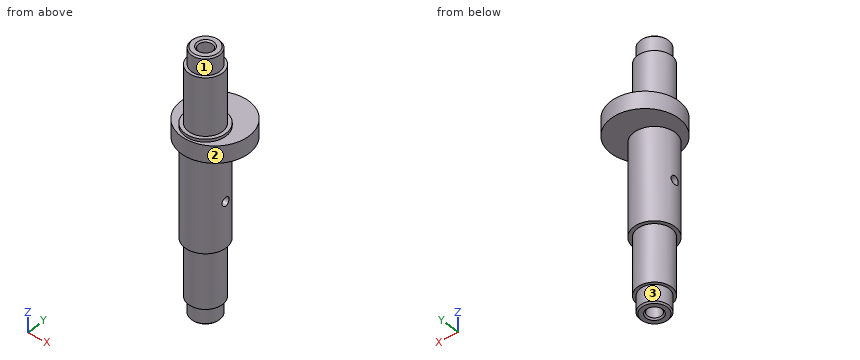
Autodesk Inventor part; units mm, degrees
ref_plane "YZ Plane" through (0, 0, 0) normal (1, 0, 0) x (0, 1, 0)
ref_plane "XZ Plane" through (0, 0, 0) normal (0, 1, 0) x (-1, 0, 0)
ref_plane "XY Plane" through (0, 0, 0) normal (0, 0, 1) x (1, 0, 0)
sketch "Sketch1" plane through (0, 0, 0) normal (0, 0, 1) x (1, 0, 0)
  circle A0 centre (0, 0) radius 12
  dimension "d0" = 24
extrude "Extrusion1" add sketch "Sketch1" along normal blind 92.4
sketch "Sketch2" plane through (0, 0, 92.4) normal (0, 0, 1) x (1, 0, 0)
  circle A0 centre (0, 0) radius 12
  circle A1 centre (0, 0) radius 5
  dimension "d3" = 10
extrude "Extrusion2" cut sketch "Sketch2" against normal blind 6.2
sketch "Sketch3" plane through (0, 0, 86.2) normal (0, 0, 1) x (1, 0, 0)
  circle A0 centre (0, 0) radius 12
  circle A1 centre (0, 0) radius 6
  dimension "d6" = 12
extrude "Extrusion3" cut sketch "Sketch3" against normal blind 20.2
sketch "Sketch4" plane through (0, 0, 66) normal (0, 0, 1) x (1, 0, 0)
  circle A0 centre (0, 0) radius 12
  circle A1 centre (0, 0) radius 7.25
  dimension "d9" = 14.5
extrude "Extrusion4" cut sketch "Sketch4" against normal blind 1
sketch "Sketch5" plane through (0, 0, 0) normal (0, 0, -1) x (-1, 0, 0)
  circle A0 centre (0, 0) radius 12
  circle A1 centre (0, 0) radius 6
  dimension "d12" = 0
  dimension "d13" = 12
extrude "Extrusion5" cut sketch "Sketch5" against normal blind 26.4
sketch "Sketch6" plane through (0, 0, 0) normal (0, 0, -1) x (-1, 0, 0)
  circle A0 centre (0, 0) radius 6
  circle A1 centre (0, 0) radius 5
  dimension "d16" = 10
extrude "Extrusion6" cut sketch "Sketch6" against normal blind 6.2
sketch "Sketch7" plane through (0, 0, 26.4) normal (0, 0, -1) x (-1, 0, 0)
  circle A0 centre (0, 0) radius 6
  circle A1 centre (0, 0) radius 12
  circle A2 centre (0, 0) radius 7.25
  dimension "d19" = 14.5
extrude "Extrusion7" cut sketch "Sketch7" against normal blind 32.6 contours A1
sketch "Sketch8" plane through (0, 0, 0) normal (0, 0, -1) x (-1, 0, 0)
  circle A0 centre (0, 0) radius 5
hole "Hole1" at (0, 0, 0) direction (0, 0, 1) diameter 4.917 depth 18 tip angle 118
chamfer "Chamfer1" distance 0.5 angle 45 1 edges at (0, -2.4585, 0)
sketch "Sketch9" plane through (0, 0, 92.4) normal (0, 0, 1) x (1, 0, 0)
  circle A0 centre (0, 0) radius 5
hole "Hole2" at (0, 0, 92.4) direction (0, 0, -1) diameter 4.917 depth 18 tip angle 118
chamfer "Chamfer2" distance 0.5 angle 45 1 edges at (0, 2.4585, 92.4)
chamfer "Chamfer3" distance 0.5 angle 45 2 edges at (-5, 0, 92.4) (5, 0, 0)
sketch "Sketch10" plane through (0, 0, 65) normal (0, 0, 1) x (1, 0, 0)
  circle A0 centre (0, 0) radius 7.25
  circle A1 centre (0, 4) radius 12
  dimension "d46" = 24
  dimension "d47" = 4
extrude "Extrusion8" add sketch "Sketch10" against normal blind 6
sketch "Sketch11" plane through (0, 0, 65) normal (0, 0, 1) x (1, 0, 0)
  arc A0 (-11.8322, 2) -> (11.8322, 2) centre (0, 0) ccw
  arc A1 (11.8322, 2) -> (-11.8322, 2) centre (0, 4) ccw
  circle A2 centre (0, 4) radius 12
extrude "Extrusion9" cut sketch "Sketch11" against normal blind 6 contours A2 A0
sketch "Sketch13" plane through (0, 0, 0) normal (1, 0, 0) x (0, 1, 0)
  circle A0 centre (0, 42.45) radius 1.5
  line L0 (-8, 59) -> (16, 59)
  line L1 (-7.25, 59) -> (7.25, 59)
  line L2 (-7.25, 26.4) -> (7.25, 26.4)
  point P0 (0, 0)
  dimension "d56" = 3
  dimension "d57" = 16.55
extrude "Extrusion11" cut sketch "Sketch13" along normal mid plane 20
properties part number "EIXO EXCÊNTRICO(53)" material "Carbon Steel"
Part model, mm, in its own coordinate system. Face numbers are marked on the shaded views. A direction names the side the tool comes from. Coordinates: 2 decimals unless noted, no trailing zeros. Loops run counter-clockwise (first coordinate to the right, second up) from the corner with the lowest first, then second, coordinate; pieces in that order, holes last. Notation, with made-up numbers: M 29.5,40.5 L 42.5,40.5 A28 cw 42.5,68.5 Z; hole C 55,-37.5 d9. An arc over 180 degrees is marked long. Use a Markdown table: item, result. Add a question column.
Q1. Pin check, flat tips, straight feed: P1, Ø2, axis at y = 4.5, z = 78, coming from the +X side; P2, Ø3, axis at x = -8, y = 8, coming from the -Z side; P3, Ø3.5, axis at y = 0, z = 42.45, coming from the +X side. Stop position of each tip, or through.
Q2. Probe L1, parallel to Y at x = 0, z = 9; L2, parallel to Z at x = -5.5, y = 10; L3, parallel to Y at x = -0.25, z = 42.45. List the from-to ranges inside material, lowest first.
Q3. Cut at B-B (z = 14.5). Write the cut outline in (x, y).
Q4. Which spindle directions (+Z, -Z, +X, -X, +Y, -Y) get a long thin tool onto all of the face, cutting with end or side? Do the marked faces 1, 2 and 3. Say none if no direction does.
Q5. Cut at A-A (z = 49.5). Write the cut outline in (x, y).
Q6. Cut at C-C (x = -8.25). Write the cut outline in (y, z).
Q7. Cut at D-D (y = 9.5). Write the cut outline in (x, z).
Worked out:
| question | item | result |
|---|---|---|
| 1 | P1 | stops at x = 4.87 |
| 1 | P2 | stops at z = 59 |
| 1 | P3 | stops at x = 7.25 |
| 2 | L1 | y = -6 to -2.46, 2.46 to 6 |
| 2 | L2 | z = 59 to 65 |
| 2 | L3 | y = -7.25 to -1.5, 1.5 to 7.25 |
| 3 | outline | C 0,0 d12; hole C 0,0 d4.92 |
| 4 | face 1 | +Z |
| 4 | face 2 | +Z, -Z |
| 4 | face 3 | -Z |
| 5 | outline | C 0,0 d14.5 |
| 6 | outline | M -4.71,59 L 12.71,59 L 12.71,65 L -4.71,65 Z |
| 7 | outline | M -10.67,59 L 10.67,59 L 10.67,65 L -10.67,65 Z |
